```python
from build123d import *

# Parameters (mm, degrees)
EXTRUDE_1_DEPTH     = 47
SKETCH_2_W          = 47
SKETCH_2_H          = 20
EXTRUDE_2_DEPTH     = 10
SKETCH_3_W          = 20
SKETCH_3_H          = 5
EXTRUDE_3_DEPTH     = 47
SKETCH_4_W          = 20
SKETCH_4_H          = 5
CUT_EXTRUDE_1_DEPTH = 99.239503256
SKETCH_5_R          = 2.05
CUT_EXTRUDE_2_DEPTH = 10
SKETCH_6_R          = 2.05
CUT_EXTRUDE_3_DEPTH = 10
SKETCH_7_W          = 1.5
SKETCH_7_H          = 7
CUT_EXTRUDE_4_DEPTH = 5
SKETCH_8_W          = 1.5
SKETCH_8_H          = 7
CUT_EXTRUDE_5_DEPTH = 5
SKETCH_9_W          = 1.8
SKETCH_9_H          = 7
CUT_EXTRUDE_6_DEPTH = 6


with BuildPart() as part:
    # 草图1 → 凸台-拉伸1 (new body)
    with BuildSketch(Plane.XY):
        with BuildLine():
            Line((0, 36), (0, 51))
            Line((0, 51), (-49, 51))
            Line((-49, 51), (-49, -51))
            Line((-49, -51), (0, -51))
            Line((0, -51), (0, -36))
            ThreePointArc((0, -36), (-36, 0), (0, 36))
        make_face()
    extrude(amount=EXTRUDE_1_DEPTH)

    # 草图2 → 凸台-拉伸2 (add)
    with BuildSketch(Plane(origin=(-10, 0, 0), x_dir=(0, 0, -1), z_dir=(1, 0, 0))):
        with Locations((-23.5, -61)):
            Rectangle(SKETCH_2_W, SKETCH_2_H)
        with Locations((-23.5, 61)):
            Rectangle(SKETCH_2_W, SKETCH_2_H)
    extrude(amount=EXTRUDE_2_DEPTH)

    # 草图3 → 凸台-拉伸3 (add, through all)
    with BuildSketch(Plane.XY.offset(47)):
        with Locations((10, 43.5)):
            Rectangle(SKETCH_3_W, SKETCH_3_H)
    extrude(amount=-EXTRUDE_3_DEPTH)

    # 草图4 → 切除-拉伸1 (cut, through all)
    with BuildSketch(Plane.XY.offset(47)):
        with Locations((-10, -43.5)):
            Rectangle(SKETCH_4_W, SKETCH_4_H)
    extrude(amount=-CUT_EXTRUDE_1_DEPTH, mode=Mode.SUBTRACT)

    # 草图5 → 切除-拉伸2 (cut)
    with BuildSketch(Plane.ZY.offset(10)):
        with Locations((10, -56)):
            Circle(SKETCH_5_R)
        with Locations((37, -56)):
            Circle(SKETCH_5_R)
    extrude(amount=-CUT_EXTRUDE_2_DEPTH, mode=Mode.SUBTRACT)

    # 草图6 → 切除-拉伸3 (cut)
    with BuildSketch(Plane.ZY.offset(10)):
        with Locations((10, 56)):
            Circle(SKETCH_6_R)
        with Locations((37, 56)):
            Circle(SKETCH_6_R)
    extrude(amount=-CUT_EXTRUDE_3_DEPTH, mode=Mode.SUBTRACT)

    # 草图7 → 切除-拉伸4 (cut)
    with BuildSketch(Plane.XZ.offset(71)):
        with Locations((-0.75, 23.5)):
            Rectangle(SKETCH_7_W, SKETCH_7_H)
    extrude(amount=-CUT_EXTRUDE_4_DEPTH, mode=Mode.SUBTRACT)

    # 草图8 → 切除-拉伸5 (cut)
    with BuildSketch(Plane(origin=(0, 71, 0), x_dir=(1, 0, 0), z_dir=(0, 1, 0))):
        with Locations((-0.75, -23.5)):
            Rectangle(SKETCH_8_W, SKETCH_8_H)
    extrude(amount=-CUT_EXTRUDE_5_DEPTH, mode=Mode.SUBTRACT)

    # 草图9 → 切除-拉伸6 (cut)
    with BuildSketch(Plane.ZY.offset(49)):
        with Locations((0.9, 0)):
            Rectangle(SKETCH_9_W, SKETCH_9_H)
    extrude(amount=-CUT_EXTRUDE_6_DEPTH, mode=Mode.SUBTRACT)


solid = part.part
```
The listing builds one solid part. Answer for the finished solid, in the listing's coordinates (mm). A direction names the side the tool comes from. Give positions to 0.01 mm unless a question says otherwise; leave off trailing zeros. Order: outer loops, then holes, each group sorted by start corner. A loop starts at its lowest first (then second) coordinate and runs counter-clockwise, first axis right, second up. Notation, with made-up numbers: (70.25, -39.5) -> (103.25, -39.5) arc R14 cw to (103.25, -17.5) -> close; hole circle Ø2 at (51, -15.5). An arc over 180 degrees is marked (long way). Answer as a JSON object with one key per item and string values. Group by question number.
Item 1: Consider L1, parallel to Y at x = -14, z = 15; L2, parallel to Y at x = -6, z = 10; L3, parallel to Y at x = -3, z = 10. Determine where each line is inside the solid, lowest interval first. Write a range as from..to.
Item 2: The part is cut by section B-B on y = -56. Write down the section's boundary in (x, z), and give its area (3 significant figures).
Item 3: The part is cut by section D-D on x = -27. Write down the section's boundary in (y, z).
Item 4: The part is cut by section A-A on z = 37. Write down the section's boundary in (x, y).
Item 5: Determine the mould class of faces 4 (the flat face through (-1.5, -69, 23)), 5 (the flat face through (-29, 51, 23)), 6 (the flat face through (-35, 10, 47)) for opening direction Z: pulls with the +Z half, pulls with the -Z half, needs draft (parallel to the pull), parting line crosses it, or undercut.
Item 6: The part is cut by section C-C on z = 14.5. Write down the section's boundary in (x, y), and give its area (3 significant figures).
Item 7: A tool of negligible diameter and unlimited length cuts with its end or side. For faces 1 (the flat face through (10, 46, 24)), 2 (the flat face through (-46, 0, 1.8)), 3 (the flat face through (0, -38, 24)), from which of +Z, -Z, +X, -X, +Y, -Y can it reach the whole face along a straight path? Write none if from no direction.
Item 8: Flat-ended cylindrical pins translate along their axes: pin 1 (0.8 mm diameter, centred on x = -1, z = 25, fed in from -Y); pin 2 (1.8 mm diameter, centred on x = -47.5, y = -1.5, fed in from -Z); pin 3 (1.5 mm diameter, centred on y = 38.5, z = 13.5, fed in from +X). Find the tip coordinate at first contact, or state that the pin passes through.
Result set:
{
 "1": {"L1": "-51..-46, -41..-33.17, 33.17..51", "L2": "-71..-58.05, -53.95..-46, -41..-35.5, 35.5..53.95, 58.05..71", "L3": "-71..-58.05, -53.95..-46, -41..-35.87, 35.87..53.95, 58.05..71"},
 "2": {"outline": "(-10, 0) -> (0, 0) -> (0, 7.95) -> (-10, 7.95) -> close; (-10, 12.05) -> (0, 12.05) -> (0, 34.95) -> (-10, 34.95) -> close; (-10, 39.05) -> (0, 39.05) -> (0, 47) -> (-10, 47) -> close", "area": "388 mm²"},
 "3": {"outline": "(-51, 0) -> (-23.81, 0) -> (-23.81, 47) -> (-51, 47) -> close; (23.81, 0) -> (51, 0) -> (51, 47) -> (23.81, 47) -> close"},
 "4": {"outline": "(-49, -51) -> (-10, -51) -> (-10, -53.95) -> (0, -53.95) -> (0, -46) -> (-20, -46) -> (-20, -41) -> (0, -41) -> (0, -36) arc R36 cw to (0, 36) -> (0, 41) -> (20, 41) -> (20, 46) -> (0, 46) -> (0, 53.95) -> (-10, 53.95) -> (-10, 51) -> (-49, 51) -> close; (-10, -71) -> (0, -71) -> (0, -58.05) -> (-10, -58.05) -> close; (-10, 58.05) -> (0, 58.05) -> (0, 71) -> (-10, 71) -> close"},
 "5": {"face 4": "undercut", "face 5": "needs draft", "face 6": "pulls with the +Z half"},
 "6": {"outline": "(-49, -51) -> (-10, -51) -> (-10, -71) -> (0, -71) -> (0, -46) -> (-20, -46) -> (-20, -41) -> (0, -41) -> (0, -36) arc R36 cw to (0, 36) -> (0, 41) -> (20, 41) -> (20, 46) -> (0, 46) -> (0, 71) -> (-10, 71) -> (-10, 51) -> (-49, 51) -> close", "area": "3,360 mm²"},
 "7": {"face 1": "+Z, -Z, +X, +Y", "face 2": "-Z, -X", "face 3": "+Z, -Z, +X, -Y"},
 "8": {"pin 1": "y = -66", "pin 2": "z = 1.8", "pin 3": "x = 0"}
}
